Geometry: see drawing. Coordinates: mm, zero at the bounding-box minimum. Give positions to 0.01 mm unless a question says otherwise; leave off trailing zeros. Write each loop counter-clockwise with the first axis right and the second up, starting at its lowest first coordinate (ties: lowest second). Pieces come first, ordered by that corner, then holes.
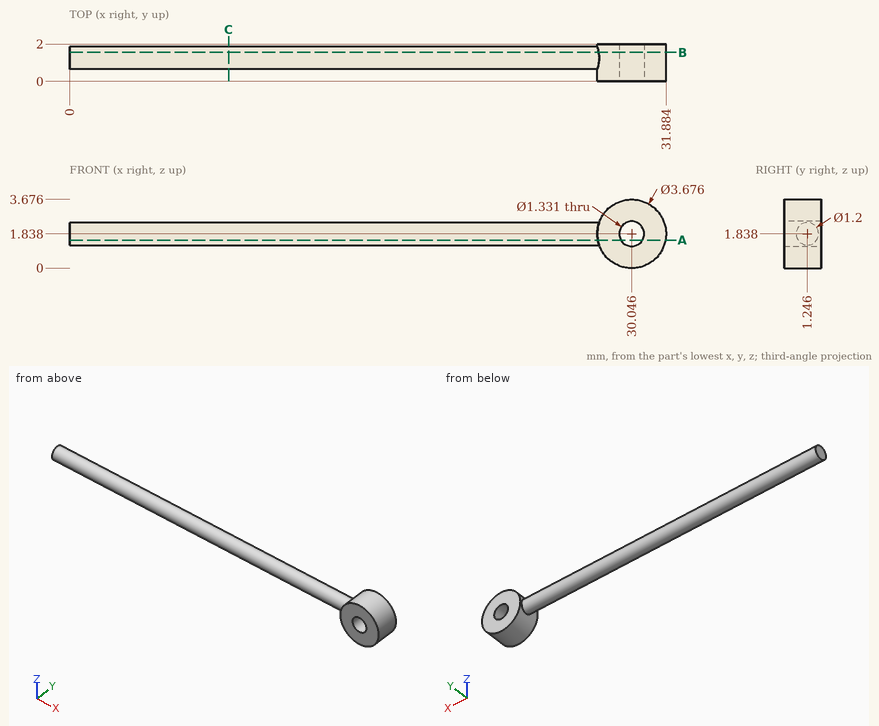
1. Pin query (flat end, axial travel): P1, Ø2, axis at x = 22.5, z = 1.5, coming from the +Y side. Return the tip coordinate at first contact, or that it passes through.
2. Section query C-C (x = 8.5). Return loops of the section in (y, z) (1 decimal), plus the area to 3 significant figures.
3. Section query A-A (z = 1.5). Return loops of the section in (x, y).
4. Line query: probe 1 along X at (y, z) = (0.7, 1.9); probe 2 along Y at (x, z) = (12.5, 1.75); probe 3 along X at (y, z) = (1.9, 2.1) (1 decimal). Output: solid intervals per line, ascending.
5. Section query B-B (y = 1.55). Return loops of the section in (x, z) (1 decimal).
The answers:
1. P1: stops at y = 1.85
2. outline: circle Ø1.2 at (1.2, 1.8)
2. area: 1.13 mm2
3. outline: (0, 0.75) - (28.24, 0.75) - (28.24, 0) - (29.47, 0) - (29.47, 2) - (28.24, 2) - (28.24, 1.74) - (0, 1.74) - close; (30.62, 0) - (31.85, 0) - (31.85, 2) - (30.62, 2) - close
4. probe 1: x = 0 to 29.38, 30.71 to 31.88
4. probe 2: y = 0.65 to 1.84
4. probe 3: x = 28.2 to 29.4, 30.7 to 31.9
5. outline: (0, 1.3) - (28.3, 1.3) arc R1.8 ccw (long way) to (28.3, 2.4) - (0, 2.4) - close; hole circle Ø1.3 at (30, 1.8)
